```python
from build123d import *

# Parameters (mm, degrees)
F0_R           = 47.625
F0_R_2         = 18
F1_DEPTH       = 6.35
F2_R           = 32.5
F3_DEPTH       = 2.5
F5_D           = 3.2
F5_DEPTH       = 10
F5_TIP         = 0.9613769904
F7_D           = 6.7564
F7_CBORE_D     = 11.1125
F7_CBORE_DEPTH = 6.35
F9_R           = 2.413
F10_DEPTH      = 16.002
F11_SIZE       = 2.286
F13_COUNT      = 3
F13_ANGLE      = 240


with BuildPart() as f1:
    # F0 (on Right) → F1 (new body, symmetric)
    with BuildSketch(Plane.YZ):
        Circle(F0_R)
        Circle(F0_R_2, mode=Mode.SUBTRACT)
    extrude(amount=F1_DEPTH, both=True)

    # F2 (on face) → F3 (cut)
    with BuildSketch(Plane.YZ.offset(6.35)):
        Circle(F2_R)
    extrude(amount=-F3_DEPTH, mode=Mode.SUBTRACT)

    # F5
    with Locations(Plane.YZ.offset(6.35)):
        with Locations((-35.814, 13.03522997), (35.814, 13.03522997), (35.814, -13.03522997), (-35.814, -13.03522997)):
            Hole(F5_D / 2, depth=F5_DEPTH)
            with Locations((0, 0, -(F5_DEPTH + F5_TIP / 2))):  # 118° drill point
                Cone(0, F5_D / 2, F5_TIP, mode=Mode.SUBTRACT)

    # F7 (through all)
    with Locations(Plane.YZ.offset(6.35)):
        with Locations((-12.7, 38.1), (12.7, 38.1), (-12.7, -38.1), (12.7, -38.1)):
            CounterBoreHole(F7_D / 2, F7_CBORE_D / 2, F7_CBORE_DEPTH)


with BuildPart() as f10:
    # F9 (on offset) → F10 (new body, symmetric)
    with BuildSketch(Plane.XY.offset(47.625)):
        Circle(F9_R)
    extrude(amount=F10_DEPTH, both=True)

    # F11
    f11_edges = [f10.edges().sort_by_distance(p)[0] for p in [
        (-2.413, 0, 31.623),
    ]]
    chamfer(f11_edges, length=F11_SIZE)


with BuildPart() as f13_1:
    # F13: instance of F10
    add(f10.part.rotate(Axis((0.1950263977, 0, 0), (1, 0, 0)), 1 * F13_ANGLE / (F13_COUNT - 1)))


with BuildPart() as f13_2:
    # F13: instance of F10
    add(f10.part.rotate(Axis((0.1950263977, 0, 0), (1, 0, 0)), 2 * F13_ANGLE / (F13_COUNT - 1)))


with BuildPart() as f1_1:
    add(f1.part)

    # F14: cut F10, F13_1, F13_2
    add(f10.part, mode=Mode.SUBTRACT)
    add(f13_1.part, mode=Mode.SUBTRACT)
    add(f13_2.part, mode=Mode.SUBTRACT)


solid = f1_1.part
```
Can you work these out from the model? Positions are in its coordinate system, mm. A direction names the side the tool comes from. Round coordinates to 2 decimals unless told otherwise and drop trailing zeros. Loops run counter-clockwise (first coordinate to the right, second up) from the corner with the lowest first, then second, coordinate; pieces in that order, holes last.
Item 1: If we mould it in two halves opening along Y, with no side actions, what happens to faces 4 (the flat face through (0, 16.3, 38.2)), 5 (the flat face through (-6.35, -1, -20)), 6 (the flat face through (0, -13, -42))? For each: +Y half, -Y half, draft (parallel to the pull), parting line (faces both ways), or undercut.
Item 2: Suppose I cut it at C-C, the plane z = -38.1. Write out the boundary of the cut face in (x, y) (3 decimals), then the cut area to 3 significant figures.
Item 3: Will these pins go through, and if not, where does the flat tip stop? pin 1 Ø5 at (x, y) = (0.5, -11) entering from -Z; pin 2 Ø1.9 at (y, z) = (-35.81, -13.04) entering from +X; pin 3 Ø6.5 at (y, z) = (12.7, 38.1) entering from -X; pin 4 Ø8 at (y, z) = (-12.7, 38.1) entering from +X.
Item 4: Suppose I cut it at D-D, the plane y = -5.5. Write out the boundary of the cut face in (x, z), then the cut area to 3 significant figures.
Item 5: Suppose I cut it at B-B, the plane y = 12. Write out the boundary of the cut face in (x, z).
Item 6: Which directions (+Z, -Z, +X, -X, +Y, -Y) give clear straight access to the entire face, cutting with the end or side of a thin tool? Please do faces 1 (the cylindrical face through (-3.22, -11.97, 34.8)), 2 (the conical face through (-0.1, -28.29, -15.48)), 3 (the cylindrical face through (3.22, -17.11, -41.48)).
Item 7: Suppose I cut it at A-A, the plane z = 7. Write out the boundary of the cut face in (x, y).
Item 8: Please list where these lines run through material, in increasing order: L1, parallel to Y at x = -2, z = -36.5; L2, parallel to X at y = -32, z = -18.5; L3, parallel to Z at x = -2, y = 35.5.
Reported:
1. face 4: undercut
1. face 5: draft
1. face 6: undercut
2. outline: (-6.35, -28.575) - (6.35, -28.575) - (6.35, -18.256) - (0, -18.256) - (0, -16.078) - (-6.35, -16.078) - close; (-6.35, -9.322) - (0, -9.322) - (0, -7.144) - (6.35, -7.144) - (6.35, 7.144) - (0, 7.144) - (0, 9.322) - (-6.35, 9.322) - close; (-6.35, 16.078) - (0, 16.078) - (0, 18.256) - (6.35, 18.256) - (6.35, 28.575) - (-6.35, 28.575) - close
2. area: 499 mm2
3. pin 1: stops at z = -46.86
3. pin 2: stops at x = -4.04
3. pin 3: passes through
3. pin 4: stops at x = 0
4. outline: (-6.35, -47.31) - (6.35, -47.31) - (6.35, -32.03) - (3.85, -32.03) - (3.85, -17.14) - (-6.35, -17.14) - close; (-6.35, 17.14) - (3.85, 17.14) - (3.85, 32.03) - (6.35, 32.03) - (6.35, 47.31) - (-6.35, 47.31) - close
4. area: 692 mm2
5. outline: (-6.35, -46.09) - (6.35, -46.09) - (6.35, -43.61) - (0, -43.61) - (0, -41.4) - (-6.35, -41.4) - close; (-6.35, -34.8) - (0, -34.8) - (0, -32.59) - (6.35, -32.59) - (6.35, -30.2) - (3.85, -30.2) - (3.85, -13.42) - (-6.35, -13.42) - close; (-6.35, 13.42) - (3.85, 13.42) - (3.85, 30.2) - (6.35, 30.2) - (6.35, 32.59) - (0, 32.59) - (0, 34.8) - (-6.35, 34.8) - close; (-6.35, 41.4) - (0, 41.4) - (0, 43.61) - (6.35, 43.61) - (6.35, 46.09) - (-6.35, 46.09) - close
6. face 1: +X, -X
6. face 2: none
6. face 3: +X
7. outline: (-6.35, -47.11) - (6.35, -47.11) - (6.35, -31.74) - (3.85, -31.74) - (3.85, -16.58) - (-6.35, -16.58) - close; (-6.35, 16.58) - (3.85, 16.58) - (3.85, 31.74) - (6.35, 31.74) - (6.35, 47.11) - (-6.35, 47.11) - close
8. L1: y = -30.59 to -15.68, -9.72 to 9.72, 15.68 to 30.59
8. L2: x = -6.35 to -2.41, 2.41 to 6.35
8. L3: z = -31.75 to -22.05, -18.94 to -14.6, -11.47 to 11.47, 14.6 to 31.75
